Here's how the part is built. I have some questions about the finished solid (model axes, mm). Face numbers are marked on the shaded views. A direction names the side the tool comes from. Coordinates: 2 decimals unless noted, no trailing zeros. Write each loop counter-clockwise with the first axis right and the second up, starting at its lowest first coordinate (ties: lowest second). Pieces come first, ordered by that corner, then holes.
Item 1: Please list where these lines run through material, in increasing order: line 1 (Z direction, x = 14.5, y = -64.5); line 2 (Y direction, x = 10, z = 19); line 3 (X direction, y = -63.5, z = 20.5).
Item 2: I want a section at D-D (z = 15). Please give me the cut outline in (x, y).
Item 3: I want a section at A-A (z = 20). Please give me the cut outline in (x, y), and give its area (3 significant figures).
Item 4: I want a section at C-C (z = 26). Please give me the cut outline in (x, y).
Item 5: If we mould it in two halves opening along X, with no side actions, what happens to the marked faces 1, 2, 3 and 4? For each: pulls with the +X half, pulls with the -X half, needs draft (parallel to the pull), parting line crosses it, or undercut.
Item 6: For the marked faces 5 and 6, which set-ups out of +Z, -Z, +X, -X, +Y, -Y let a thin tool reach every point of the face, with its end or its side?
Item 7: I'm going to push flat-ended pins straight in: P1, Ø0.8, axis at x = 34, y = -65.5, coming from the +Z side; P2, Ø4, axis at x = 14, z = 17, coming from the -Y side; P3, Ø2, axis at x = 17, z = 15.5, coming from the -Y side. Where does each tip first touch, or does it pass through?
Item 8: I want a section at B-B (z = 5). Please give me the cut outline in (x, y).
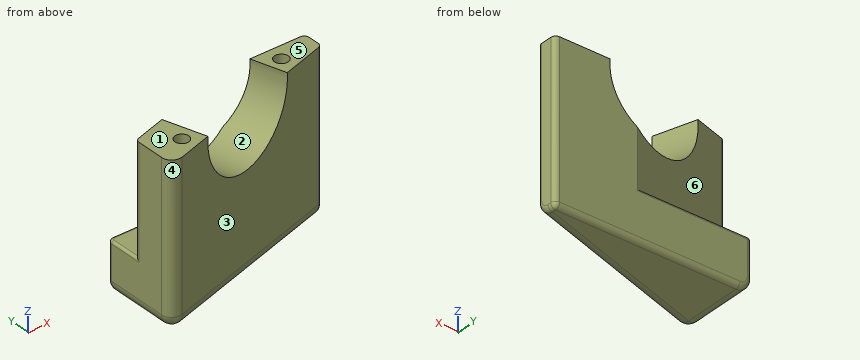
from build123d import *

# Parameters (mm, degrees)
PAD005_DEPTH      = 31
PAD005_DEPTH_BACK = 1
SKETCH005_R       = 11.2
POCKET_DEPTH      = 15.56696
POCKET006_DEPTH   = 22
SKETCH016_R       = 1.4
POCKET009_DEPTH   = 15
FILLET003_R       = 2.5
FILLET004_R       = 1
FILLET005_R       = 1
FILLET006_R       = 1
FILLET007_R       = 0.5


with BuildPart() as part:
    # Sketch004 → Pad005 (new body, two sides)
    with BuildSketch(Plane.XY) as pad005_sk:
        with BuildLine():
            Line((41.8431, -62), (1.8431, -62))
            Line((1.8431, -62), (1.8431, -75.526382))
            ThreePointArc((1.8431, -75.526382), (2.653454, -77.134096), (4.427843, -77.438992))
            Line((4.427843, -77.438992), (41.8431, -66))
            Line((41.8431, -66), (41.8431, -62))
        make_face()
    extrude(amount=PAD005_DEPTH)
    extrude(pad005_sk.sketch, amount=-PAD005_DEPTH_BACK)

    # Sketch005 → Pocket (cut, through all)
    with BuildSketch(Plane(origin=(22.043577, -72.101291, 0), x_dir=(0.956305, 0.292372, 0), z_dir=(0.292372, -0.956305, 0))):
        with Locations((0, 30)):
            Circle(SKETCH005_R)
    extrude(amount=-POCKET_DEPTH, mode=Mode.SUBTRACT)

    # Sketch007 → Pocket006 (cut)
    with BuildSketch(Plane.XY.offset(31)):
        Polygon((-4.66376, -53.953282), (-5.90948, -71.46493), (38.1328, -58.000022), (37.116007, -54.0061), align=None)
    extrude(amount=-POCKET006_DEPTH, mode=Mode.SUBTRACT)

    # Sketch016 → Pocket009 (cut)
    with BuildSketch(Plane.XY.offset(31)):
        with Locations((34.498539, -65.108382)):
            Circle(SKETCH016_R)
        with Locations((7.722005, -73.29479)):
            Circle(SKETCH016_R)
    extrude(amount=-POCKET009_DEPTH, mode=Mode.SUBTRACT)

    # Fillet003
    fillet003_edges = [part.edges().sort_by_distance(p)[0] for p in [
        (23.135472, -71.719496, -1),
    ]]
    fillet(fillet003_edges, radius=FILLET003_R)

    # Fillet004
    fillet004_edges = [part.edges().sort_by_distance(p)[0] for p in [
        (41.8431, -66, 16.25),
    ]]
    fillet(fillet004_edges, radius=FILLET004_R)

    # Fillet005
    fillet005_edges = [part.edges().sort_by_distance(p)[0] for p in [
        (41.8431, -62, 15.5),
    ]]
    fillet(fillet005_edges, radius=FILLET005_R)

    # Fillet006
    fillet006_edges = [part.edges().sort_by_distance(p)[0] for p in [
        (1.8431, -69.094758, 20),
    ]]
    fillet(fillet006_edges, radius=FILLET006_R)

    # Fillet007
    fillet007_edges = [part.edges().sort_by_distance(p)[0] for p in [
        (1.8431, -66.047379, 9),
    ]]
    fillet(fillet007_edges, radius=FILLET007_R)


solid = part.part
Answer:
1. line 1: z = -1 to 9
1. line 2: y = -75.74 to -66.6
1. line 3: x = 25.62 to 41.84
2. outline: (1.84, -75.53) arc R2 ccw to (4.43, -77.44) - (41.14, -66.22) arc R1 ccw to (41.84, -65.26) - (41.84, -63) arc R1 ccw to (40.84, -62) - (25.05, -62) - (2.55, -68.88) arc R1 ccw to (1.84, -69.83) - close
3. outline: (1.84, -75.53) arc R2 ccw to (4.43, -77.44) - (17.21, -73.53) - (14.65, -65.18) - (2.55, -68.88) arc R1 ccw to (1.84, -69.83) - close; (24.3, -62.23) - (26.85, -70.58) - (41.14, -66.22) arc R1 ccw to (41.84, -65.26) - (41.84, -63) arc R1 ccw to (40.84, -62) - (25.05, -62) - close; hole circle Ø2.8 at (7.72, -73.29); hole circle Ø2.8 at (34.5, -65.11)
3. area: 220 mm2
4. outline: (1.84, -75.53) arc R2 ccw to (4.43, -77.44) - (12.03, -75.12) - (9.47, -66.76) - (2.55, -68.88) arc R1 ccw to (1.84, -69.83) - close; (29.89, -62) - (32.03, -69) - (41.14, -66.22) arc R1 ccw to (41.84, -65.26) - (41.84, -63) arc R1 ccw to (40.84, -62) - close; hole circle Ø2.8 at (7.72, -73.29); hole circle Ø2.8 at (34.5, -65.11)
5. face 1: needs draft
5. face 2: undercut
5. face 3: pulls with the +X half
5. face 4: parting line crosses it
6. face 5: +Z, +X, -X, +Y, -Y
6. face 6: +Z, -X, +Y
7. P1: stops at z = 16
7. P2: stops at y = -75.12
7. P3: stops at y = -73.9
8. outline: (1.84, -75.53) arc R2 ccw to (4.43, -77.44) - (41.14, -66.22) arc R1 ccw to (41.84, -65.26) - (41.84, -63) arc R1 ccw to (40.84, -62) - (2.84, -62) arc R1 ccw to (1.84, -63) - close
